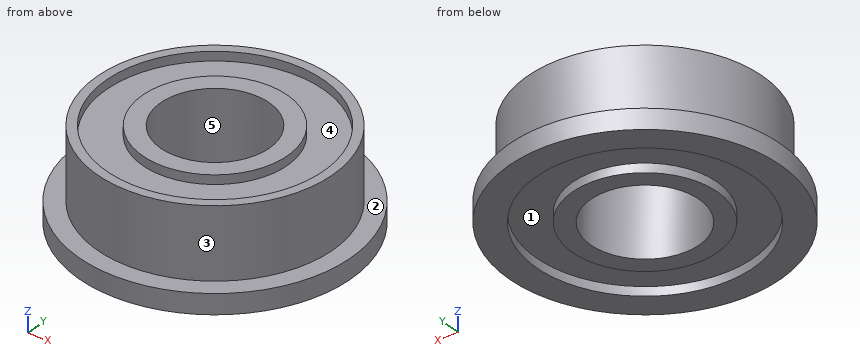
from build123d import *

# Parameters (mm, degrees)
SKETCH1_R           = 7.5
SKETCH1_R_2         = 3
BOSS_EXTRUDE1_DEPTH = 1.1
SKETCH2_R           = 6.5
SKETCH2_R_2         = 3
BOSS_EXTRUDE2_DEPTH = 3.9
SKETCH3_R           = 6
SKETCH3_R_2         = 4
CUT_EXTRUDE1_DEPTH  = 0.5


with BuildPart() as part:
    # Sketch1 → Boss-Extrude1 (new body)
    with BuildSketch(Plane.XY):
        Circle(SKETCH1_R)
        Circle(SKETCH1_R_2, mode=Mode.SUBTRACT)
    extrude(amount=BOSS_EXTRUDE1_DEPTH)

    # Sketch2 → Boss-Extrude2 (add)
    with BuildSketch(Plane.XY.offset(1.1)):
        Circle(SKETCH2_R)
        Circle(SKETCH2_R_2, mode=Mode.SUBTRACT)
    extrude(amount=BOSS_EXTRUDE2_DEPTH)

    # Sketch3 → Cut-Extrude1 (cut)
    with BuildSketch(Plane(origin=(0, 0, 0), x_dir=(-1, 0, 0), z_dir=(0, 0, -1))):
        Circle(SKETCH3_R)
        Circle(SKETCH3_R_2, mode=Mode.SUBTRACT)
    cut_extrude1 = extrude(amount=-CUT_EXTRUDE1_DEPTH, mode=Mode.SUBTRACT)

    # Mirror1: Cut-Extrude1 across plane
    add(cut_extrude1.mirror(Plane.XY.offset(2.5)), mode=Mode.SUBTRACT)


solid = part.part
Could you check a few things on this model? Use its own coordinates, in mm. Face numbers are marked on the shaded views. A direction names the side the tool comes from. Round coordinates to 2 decimals unless told otherwise and drop trailing zeros. Order: outer loops, then holes, each group sorted by start corner. A loop starts at its lowest first (then second) coordinate and runs counter-clockwise, first axis right, second up.
(1) Which directions (+Z, -Z, +X, -X, +Y, -Y) give clear straight access to the entire face, cutting with the end or side of a thin tool? Please do the marked faces 4 and 5.
Response values:
face 4: +Z
face 5: +Z, -Z
(2) I'm going to push flat-ended pins straight in: pin 1 (1 mm diameter, centred on x = -4.5, y = -1.5, fed in from -Z); pin 2 (1 mm diameter, centred on x = -1.5, z = 3, fed in from -Y); pin 3 (1 mm diameter, centred on y = -5.5, z = 3, fed in from -X). Where does each tip first touch, or does it pass through?
Response values:
pin 1: stops at z = 0.5
pin 2: stops at y = -6.42
pin 3: stops at x = -4.15
(3) Imagine slicing it at D-D (y = -3.5). Write out the boundary of the cut face in (x, z), plus the area to 3 significant figures.
Response values:
outline: (-6.63, 0) - (-4.87, 0) - (-4.87, 0.5) - (-1.94, 0.5) - (-1.94, 0) - (1.94, 0) - (1.94, 0.5) - (4.87, 0.5) - (4.87, 0) - (6.63, 0) - (6.63, 1.1) - (5.48, 1.1) - (5.48, 5) - (4.87, 5) - (4.87, 4.5) - (1.94, 4.5) - (1.94, 5) - (-1.94, 5) - (-1.94, 4.5) - (-4.87, 4.5) - (-4.87, 5) - (-5.48, 5) - (-5.48, 1.1) - (-6.63, 1.1) - close
area: 51.4 mm2
(4) Please list where these lines run through material, in increasing order: line 1 along Y through (x, z) = (0, 4.6); line 2 along Y through (x, z) = (0, 0.25); line 3 along X through (y, z) = (-3.5, 0.45).
Response values:
line 1: y = -6.5 to -6, -4 to -3, 3 to 4, 6 to 6.5
line 2: y = -7.5 to -6, -4 to -3, 3 to 4, 6 to 7.5
line 3: x = -6.63 to -4.87, -1.94 to 1.94, 4.87 to 6.63
(5) Imagine slicing it at B-B (x = 2.25). Write out the boundary of the cut face in (y, z).
Response values:
outline: (-7.15, 0) - (-5.56, 0) - (-5.56, 0.5) - (-3.31, 0.5) - (-3.31, 0) - (-1.98, 0) - (-1.98, 5) - (-3.31, 5) - (-3.31, 4.5) - (-5.56, 4.5) - (-5.56, 5) - (-6.1, 5) - (-6.1, 1.1) - (-7.15, 1.1) - close; (1.98, 0) - (3.31, 0) - (3.31, 0.5) - (5.56, 0.5) - (5.56, 0) - (7.15, 0) - (7.15, 1.1) - (6.1, 1.1) - (6.1, 5) - (5.56, 5) - (5.56, 4.5) - (3.31, 4.5) - (3.31, 5) - (1.98, 5) - close
(6) Imagine slicing it at A-A (y = 0). Write out the boundary of the cut face in (x, z), plus the area to 3 significant figures.
Response values:
outline: (-7.5, 0) - (-6, 0) - (-6, 0.5) - (-4, 0.5) - (-4, 0) - (-3, 0) - (-3, 5) - (-4, 5) - (-4, 4.5) - (-6, 4.5) - (-6, 5) - (-6.5, 5) - (-6.5, 1.1) - (-7.5, 1.1) - close; (3, 0) - (4, 0) - (4, 0.5) - (6, 0.5) - (6, 0) - (7.5, 0) - (7.5, 1.1) - (6.5, 1.1) - (6.5, 5) - (6, 5) - (6, 4.5) - (4, 4.5) - (4, 5) - (3, 5) - close
area: 33.2 mm2
(7) If we mould it in two halves opening along X, with no side actions, what happens to the marked faces 1, 2 and 3? For each: released by +X, released by -X, zero draft, split by the parting line, or undercut.
Response values:
face 1: undercut
face 2: zero draft
face 3: split by the parting line
(8) Imagine slicing it at C-C (z = 2.4). Write out the boundary of the cut face in (x, y), plus the area to 3 significant figures.
Response values:
outline: circle Ø13 at (0, 0); hole circle Ø6 at (0, 0)
area: 104 mm2
